```python
from build123d import *

# Parameters (mm, degrees)
F0_R     = 1.4
F0_W     = 4.5
F0_H     = 4.5
F1_DEPTH = 2


with BuildPart() as f1:
    # F0 (on Top) → F1 (new body)
    with BuildSketch(Plane.XY):
        with BuildLine():
            Line((71.545826, 22.863086), (-72.454174, 22.863086))
            ThreePointArc((-72.454174, 22.863086), (-73.868388, 22.277299), (-74.454174, 20.863086))
            Line((-74.454174, 20.863086), (-74.454174, -59.136914))
            ThreePointArc((-74.454174, -59.136914), (-73.868388, -60.551128), (-72.454174, -61.136914))
            Line((-72.454174, -61.136914), (71.545826, -61.136914))
            ThreePointArc((71.545826, -61.136914), (72.960039, -60.551128), (73.545826, -59.136914))
            Line((73.545826, -59.136914), (73.545826, 20.863086))
            ThreePointArc((73.545826, 20.863086), (72.960039, 22.277299), (71.545826, 22.863086))
        make_face()
        with Locations((-69.454174, -56.136914)):
            Circle(F0_R, mode=Mode.SUBTRACT)
        with Locations((-64.137191, -49.445186)):
            Rectangle(F0_W, F0_H, mode=Mode.SUBTRACT)
        with Locations((-56.137191, -49.445186)):
            Rectangle(F0_W, F0_H, mode=Mode.SUBTRACT)
        with Locations((-64.204174, -41.886914)):
            Rectangle(F0_W, F0_H, mode=Mode.SUBTRACT)
        with Locations((-56.204174, -41.886914)):
            Rectangle(F0_W, F0_H, mode=Mode.SUBTRACT)
        with Locations((-48.137191, -49.445186)):
            Rectangle(F0_W, F0_H, mode=Mode.SUBTRACT)
        with Locations((-40.137191, -49.445186)):
            Rectangle(F0_W, F0_H, mode=Mode.SUBTRACT)
        with Locations((-48.204174, -41.886914)):
            Rectangle(F0_W, F0_H, mode=Mode.SUBTRACT)
        with Locations((-40.204174, -41.886914)):
            Rectangle(F0_W, F0_H, mode=Mode.SUBTRACT)
        with Locations((-32.137191, -49.445186)):
            Rectangle(F0_W, F0_H, mode=Mode.SUBTRACT)
        with Locations((-24.137191, -49.445186)):
            Rectangle(F0_W, F0_H, mode=Mode.SUBTRACT)
        with Locations((-32.204174, -41.886914)):
            Rectangle(F0_W, F0_H, mode=Mode.SUBTRACT)
        with Locations((-24.204174, -41.886914)):
            Rectangle(F0_W, F0_H, mode=Mode.SUBTRACT)
        with Locations((-16.137191, -49.445186)):
            Rectangle(F0_W, F0_H, mode=Mode.SUBTRACT)
        with Locations((-8.137191, -49.445186)):
            Rectangle(F0_W, F0_H, mode=Mode.SUBTRACT)
        with Locations((-16.204174, -41.886914)):
            Rectangle(F0_W, F0_H, mode=Mode.SUBTRACT)
        with Locations((-8.204174, -41.886914)):
            Rectangle(F0_W, F0_H, mode=Mode.SUBTRACT)
        with Locations((-44.454174, -33.636914)):
            Circle(F0_R, mode=Mode.SUBTRACT)
        with Locations((-0.137191, -49.445186)):
            Rectangle(F0_W, F0_H, mode=Mode.SUBTRACT)
        with Locations((7.862809, -49.445186)):
            Rectangle(F0_W, F0_H, mode=Mode.SUBTRACT)
        with Locations((15.862809, -49.445186)):
            Rectangle(F0_W, F0_H, mode=Mode.SUBTRACT)
        with Locations((-0.204174, -41.886914)):
            Rectangle(F0_W, F0_H, mode=Mode.SUBTRACT)
        with Locations((7.795826, -41.886914)):
            Rectangle(F0_W, F0_H, mode=Mode.SUBTRACT)
        with Locations((15.795826, -41.886914)):
            Rectangle(F0_W, F0_H, mode=Mode.SUBTRACT)
        with Locations((23.862809, -49.445186)):
            Rectangle(F0_W, F0_H, mode=Mode.SUBTRACT)
        with Locations((31.862809, -49.445186)):
            Rectangle(F0_W, F0_H, mode=Mode.SUBTRACT)
        with Locations((23.795826, -41.886914)):
            Rectangle(F0_W, F0_H, mode=Mode.SUBTRACT)
        with Locations((31.795826, -41.886914)):
            Rectangle(F0_W, F0_H, mode=Mode.SUBTRACT)
        with Locations((44.545826, -56.136914)):
            Circle(F0_R, mode=Mode.SUBTRACT)
        with Locations((39.862809, -49.445186)):
            Rectangle(F0_W, F0_H, mode=Mode.SUBTRACT)
        with Locations((47.862809, -49.445186)):
            Rectangle(F0_W, F0_H, mode=Mode.SUBTRACT)
        with Locations((39.795826, -41.886914)):
            Rectangle(F0_W, F0_H, mode=Mode.SUBTRACT)
        with Locations((47.795826, -41.886914)):
            Rectangle(F0_W, F0_H, mode=Mode.SUBTRACT)
        with Locations((55.862809, -49.445186)):
            Rectangle(F0_W, F0_H, mode=Mode.SUBTRACT)
        with Locations((63.862809, -49.445186)):
            Rectangle(F0_W, F0_H, mode=Mode.SUBTRACT)
        with Locations((55.795826, -41.886914)):
            Rectangle(F0_W, F0_H, mode=Mode.SUBTRACT)
        with Locations((63.795826, -41.886914)):
            Rectangle(F0_W, F0_H, mode=Mode.SUBTRACT)
        with Locations((68.545826, -33.636914)):
            Circle(F0_R, mode=Mode.SUBTRACT)
        with Locations((-69.454174, 17.863086)):
            Circle(F0_R, mode=Mode.SUBTRACT)
        with Locations((-44.454174, 17.863086)):
            Circle(F0_R, mode=Mode.SUBTRACT)
        with BuildLine():
            Line((-45.954174, -30.136914), (-45.954174, 14.363086))
            Line((-45.954174, 14.363086), (-43.954174, 14.363086))
            ThreePointArc((-43.954174, 14.363086), (-41.832854, 15.241765), (-40.954174, 17.363086))
            Line((-40.954174, 17.363086), (65.045826, 17.363086))
            ThreePointArc((65.045826, 17.363086), (65.924505, 15.241765), (68.045826, 14.363086))
            Line((68.045826, 14.363086), (68.045826, -30.136914))
            ThreePointArc((68.045826, -30.136914), (65.924505, -31.015594), (65.045826, -33.136914))
            Line((65.045826, -33.136914), (65.045826, -35.136914))
            Line((65.045826, -35.136914), (-40.954174, -35.136914))
            Line((-40.954174, -35.136914), (-40.954174, -33.136914))
            ThreePointArc((-40.954174, -33.136914), (-41.832854, -31.015594), (-43.954174, -30.136914))
            Line((-43.954174, -30.136914), (-45.954174, -30.136914))
        make_face(mode=Mode.SUBTRACT)
        with Locations((68.545826, 17.863086)):
            Circle(F0_R, mode=Mode.SUBTRACT)
    extrude(amount=F1_DEPTH)


solid = f1.part
```
Design review of the part built by this model. Coordinates are the model's own, in mm. A direction names the side the tool comes from. Give positions to 0.01 mm unless a question says otherwise; leave off trailing zeros. Loops run counter-clockwise (first coordinate to the right, second up) from the corner with the lowest first, then second, coordinate; pieces in that order, holes last. Notation, with made-up numbers: (2, 79.5) -> (50, 79.5) arc R24 ccw to (50, 115.5) -> close; hole circle Ø6 at (13, 53.5). An arc over 180 degrees is marked (long way). One line per item, written item: value.
Q1. For L1, parallel to Y at x = 1, z = 0.2; L2, parallel to X at y = 8, z = 1.15; L3, parallel to Y at x = -21.5, z = 1.85, list the stretches that pass through material, from the lowest coordinate up.
Numbers:
L1: y = -61.14 to -51.7, -47.2 to -44.14, -39.64 to -35.14, 17.36 to 22.86
L2: x = -74.45 to -45.95, 68.05 to 73.55
L3: y = -61.14 to -35.14, 17.36 to 22.86
Q2. We need section C-C on x = -57. Give the boundary of the cut face in (y, z), and give its area (3 significant figures).
Numbers:
outline: (-61.14, 0) -> (-51.7, 0) -> (-51.7, 2) -> (-61.14, 2) -> close; (-47.2, 0) -> (-44.14, 0) -> (-44.14, 2) -> (-47.2, 2) -> close; (-39.64, 0) -> (22.86, 0) -> (22.86, 2) -> (-39.64, 2) -> close
area: 150 mm^2
Q3. We need section D-D on x = 55.5. Give the boundary of the cut face in (y, z).
Numbers:
outline: (-61.14, 0) -> (-51.7, 0) -> (-51.7, 2) -> (-61.14, 2) -> close; (-47.2, 0) -> (-44.14, 0) -> (-44.14, 2) -> (-47.2, 2) -> close; (-39.64, 0) -> (-35.14, 0) -> (-35.14, 2) -> (-39.64, 2) -> close; (17.36, 0) -> (22.86, 0) -> (22.86, 2) -> (17.36, 2) -> close
Q4. We need section A-A on x = 4. Give the boundary of the cut face in (y, z), and give its area (3 significant figures).
Numbers:
outline: (-61.14, 0) -> (-35.14, 0) -> (-35.14, 2) -> (-61.14, 2) -> close; (17.36, 0) -> (22.86, 0) -> (22.86, 2) -> (17.36, 2) -> close
area: 63.0 mm^2
Q5. Draft analysis for pull direction X (two halves, no side actions). For faces 3 (the cylindrical face through (-41.856, 15.219, 0.986)), 4 (the cylindrical face through (43.147, -56.075, 0.986)), 5 (the flat face through (-18, -37, 2)), state which applies: pulls with the +X half, pulls with the -X half, needs draft (parallel to the pull), parting line crosses it, or undercut.
Numbers:
face 3: undercut
face 4: undercut
face 5: needs draft
Q6. Machinability: for faces 1 (the flat face through (-18, -37, 0)), 2 (the cylindrical face through (-41.81, -31.04, 0.99)), which of the approach directions +Z, -Z, +X, -X, +Y, -Y give a long, thin tool a straight path to every point of the face, cutting with its end or side? Answer none if there is none.
Numbers:
face 1: -Z, +X, -X, +Y, -Y
face 2: +Z, -Z
Q7. We need section B-B on y = 2.5. Give the boundary of the cut face in (x, z), and give its area (3 significant figures).
Numbers:
outline: (-74.45, 0) -> (-45.95, 0) -> (-45.95, 2) -> (-74.45, 2) -> close; (68.05, 0) -> (73.55, 0) -> (73.55, 2) -> (68.05, 2) -> close
area: 68.0 mm^2
